Part model, mm, in its own coordinate system. Face numbers are marked on the shaded views. A direction names the side the tool comes from. Coordinates: 2 decimals unless noted, no trailing zeros. Loops run counter-clockwise (first coordinate to the right, second up) from the corner with the lowest first, then second, coordinate; pieces in that order, holes last. Notation, with made-up numbers: M 30,19.25 L 61,19.25 A25 ccw 61,42.25 Z; hole C -12,31.5 d5. An arc over 180 degrees is marked long. Answer as CSV lines item,"result". Start each with the question number.
Autodesk Inventor part; units mm, degrees
ref_plane "YZ Plane" through (0, 0, 0) normal (1, 0, 0) x (0, 1, 0)
ref_plane "XZ Plane" through (0, 0, 0) normal (0, 1, 0) x (-1, 0, 0)
ref_plane "XY Plane" through (0, 0, 0) normal (0, 0, 1) x (1, 0, 0)
sketch "Sketch1" plane through (0, 0, 0) normal (0, 0, 1) x (1, 0, 0)
  line L0 (-107.95, 107.95) -> (107.95, 107.95)
  line L1 (107.95, 107.95) -> (107.95, -107.95)
  line L2 (107.95, -107.95) -> (-107.95, -107.95)
  line L3 (-107.95, -107.95) -> (-107.95, 107.95)
  line L4 (-107.95, -107.95) -> (107.95, 107.95) construction
  point P0 (0, 0)
  point P1 (0, 0)
  dimension "d0" = 215.9
  dimension "d1" = 215.9
extrude "Extrusion1" add sketch "Sketch1" along normal blind 3
sketch "Sketch3" plane through (0, 0, 0) normal (0, 0, -1) x (-1, 0, 0)
  line L0 (256.032, 0) -> (-256.032, 0) construction
  line L1 (0, -256.032) -> (0, 256.032) construction
  line L2 (-101.6, 101.6) -> (101.6, 101.6) construction
  line L3 (-101.6, -101.6) -> (101.6, -101.6) construction
  line L4 (101.6, 101.6) -> (-101.6, -101.6) construction
  line L5 (101.6, -101.6) -> (-101.6, 101.6) construction
  arc A0 (-90.3175, 92.5625) -> (-92.5625, 92.5625) centre (-91.44, 91.44) ccw
  arc A1 (-90.3175, 92.5625) -> (0, 55.1518) centre (0, 182.88) ccw
  line L6 (-91.44, 91.44) -> (0, 182.88) construction
  arc A2 (-92.5625, 92.5625) -> (-92.5625, 90.3175) centre (-91.44, 91.44) ccw
  arc A3 (-55.1518, 0) -> (-92.5625, 90.3175) centre (-182.88, 0) ccw
  arc A4 (92.5625, 92.5625) -> (90.3175, 92.5625) centre (91.44, 91.44) ccw
  arc A5 (0, 55.1518) -> (90.3175, 92.5625) centre (0, 182.88) ccw
  arc A6 (92.5625, 90.3175) -> (55.1518, 0) centre (182.88, 0) ccw
  arc A7 (92.5625, 90.3175) -> (92.5625, 92.5625) centre (91.44, 91.44) ccw
  arc A8 (-92.5625, -92.5625) -> (-90.3175, -92.5625) centre (-91.44, -91.44) ccw
  arc A9 (0, -55.1518) -> (-90.3175, -92.5625) centre (0, -182.88) ccw
  arc A10 (-92.5625, -90.3175) -> (-55.1518, 0) centre (-182.88, 0) ccw
  arc A11 (-92.5625, -90.3175) -> (-92.5625, -92.5625) centre (-91.44, -91.44) ccw
  arc A12 (55.1518, 0) -> (92.5625, -90.3175) centre (182.88, 0) ccw
  arc A13 (90.3175, -92.5625) -> (0, -55.1518) centre (0, -182.88) ccw
  arc A14 (90.3175, -92.5625) -> (92.5625, -92.5625) centre (91.44, -91.44) ccw
  arc A15 (92.5625, -92.5625) -> (92.5625, -90.3175) centre (91.44, -91.44) ccw
  point P0 (0, 0)
  dimension "d168" = 3.175
  dimension "d169" = 91.44
extrude "Extrusion5" cut sketch "Sketch3" against normal blind 0.7
sketch "Sketch6" plane through (0, 0, 0.7) normal (0, 0, -1) x (-1, 0, 0)
  circle A0 centre (0, 0) radius 55.1518
  arc A1 (-90.3175, 92.5625) -> (-92.5625, 90.3175) centre (-91.44, 91.44) ccw
  arc A2 (-92.5625, -90.3175) -> (-92.5625, 90.3175) centre (-182.88, 0) ccw
  arc A3 (-92.5625, -90.3175) -> (-90.3175, -92.5625) centre (-91.44, -91.44) ccw
  arc A4 (90.3175, -92.5625) -> (-90.3175, -92.5625) centre (0, -182.88) ccw
  arc A5 (90.3175, -92.5625) -> (92.5625, -90.3175) centre (91.44, -91.44) ccw
  arc A6 (92.5625, 90.3175) -> (92.5625, -90.3175) centre (182.88, 0) ccw
  arc A7 (92.5625, 90.3175) -> (90.3175, 92.5625) centre (91.44, 91.44) ccw
  arc A8 (-90.3175, 92.5625) -> (90.3175, 92.5625) centre (0, 182.88) ccw
  arc A9 (-90.3175, 92.5625) -> (90.3175, 92.5625) centre (0, 182.88) ccw
  point P0 (0, 0)
extrude "Extrusion6" cut sketch "Sketch6" against normal up to next contours A0
sketch "Sketch11" plane through (0, 0, 3) normal (0, 0, 1) x (1, 0, 0)
  line L0 (-91.44, 91.44) -> (91.44, 91.44) construction
  line L1 (91.44, 91.44) -> (91.44, -91.44) construction
  line L2 (91.44, -91.44) -> (-91.44, -91.44) construction
  line L3 (-91.44, -91.44) -> (-91.44, 91.44) construction
  line L4 (-151.13, 0) -> (151.13, 0) construction
  line L5 (0, -151.13) -> (0, 151.13) construction
  point P0 (0, 0)
  dimension "d170" = 182.88
  dimension "d171" = 182.88
hole "Hole15" at (-91.44, 91.44, 3) at (91.44, 91.44, 3) at (91.44, -91.44, 3) at (-91.44, -91.44, 3) direction (0, 0, -1) diameter 3.175 end through all
sketch "Sketch13" plane through (0, 0, 3) normal (0, 0, 1) x (1, 0, 0)
  line L0 (-91.44, -91.44) -> (91.44, -91.44) construction
  line L1 (91.44, -91.44) -> (91.44, 91.44) construction
  line L2 (91.44, 91.44) -> (-91.44, 91.44) construction
  line L3 (-91.44, 91.44) -> (-91.44, -91.44) construction
  line L4 (-91.44, -91.44) -> (91.44, 91.44) construction
  line L5 (-151.13, 0) -> (151.13, 0) construction
  line L6 (0, -151.13) -> (0, 151.13) construction
  point P0 (0, 0)
  point P1 (0, 0)
  point P2 (-68.58, 91.44)
  point P3 (0, 91.44)
  point P4 (68.58, 91.44)
  point P5 (91.44, 68.58)
  point P6 (91.44, 0)
  point P7 (91.44, -68.58)
  point P8 (68.58, -91.44)
  point P9 (0, -91.44)
  point P10 (-68.58, -91.44)
  point P11 (-91.44, -68.58)
  point P12 (-91.44, 0)
  point P13 (-91.44, 68.58)
  dimension "d302" = 182.88
  dimension "d303" = 182.88
  dimension "d304" = 22.86
  dimension "d305" = 22.86
hole "Hole29" at (-68.58, 91.44, 3) at (0, 91.44, 3) at (68.58, 91.44, 3) at (91.44, 68.58, 3) at (91.44, 0, 3) at (91.44, -68.58, 3) at (68.58, -91.44, 3) at (0, -91.44, 3) at (-68.58, -91.44, 3) at (-91.44, -68.58, 3) at (-91.44, 0, 3) at (-91.44, 68.58, 3) direction (0, 0, -1) diameter 4.4958 end through all
sketch "Sketch14" plane through (0, 0, 3) normal (0, 0, 1) x (1, 0, 0)
  circle A0 centre (0, 0) radius 55.1518
  line L0 (0, -151.13) -> (0, 151.13) construction
  circle A1 centre (0, 55.1518) radius 1.5875
  point P0 (0, 0)
  dimension "d313" = 3.175
extrude "Extrusion9" cut sketch "Sketch14" against normal through all contours A1 A0 | A0 A1 picked at (0.0632, 54.6247) picked at (0.0603, 55.6758)
equation "\"d1\" = d0"
properties part number "J002446_1" material "UHMW, WHITE"
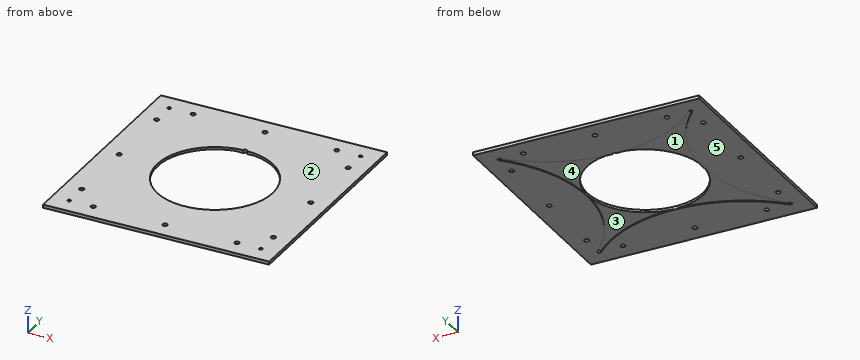
Q1. Slice it at B-B, the plane x = -10. Write the cut outline in (y, z).
Q2. Slice it at C-C, the plane x = 21. Write the cut outline in (y, z), and give its area (3 significant figures).
Q3. Two-plate mould, pull along X, no slides. Class the marked faces 3, 4 and 5: +X half, -X half, draft (parallel to the pull), parting line (faces both ways), or undercut.
Q4. Slice it at A-A, the plane z = 2.1. State how many separate pieces and enclosed holes the cut face has, and give its area (3 significant figures).
Q5. Tool access for the marked faces 1 and 2: list every direction of +Z, -Z, +X, -X, +Y, -Y with a clear straight run to the whole face (end or side of a thin tool).
Q6. Wall check: L1, parallel to X at y = 0, z = 1.1; L2, parallel to X at y = 91.44, z = 2.15. Give the ranges that are in metal, low to high.
Solved:
1,outline,"M -107.95,0 L -55.54,0 L -55.54,0.7 L -54.24,0.7 L -54.24,3 L -107.95,3 Z; M 54.24,0.7 L 55.54,0.7 L 55.54,0 L 107.95,0 L 107.95,3 L 54.24,3 Z"
2,outline,"M -107.95,0 L -56.89,0 L -56.89,0.7 L -51,0.7 L -51,3 L -107.95,3 Z; M 51,0.7 L 56.89,0.7 L 56.89,0 L 107.95,0 L 107.95,3 L 51,3 Z"
2,area,"333 mm2"
3,face 3,"undercut"
3,face 4,"undercut"
3,face 5,"draft"
4,separate pieces,"1"
4,enclosed holes,"17"
4,area,"36,800 mm2"
5,face 1,"-Z"
5,face 2,"+Z, +X, -X, +Y, -Y"
6,L1,"x = -107.95 to -93.69, -89.19 to -55.15, 55.15 to 89.19, 93.69 to 107.95"
6,L2,"x = -107.95 to -93.03, -89.85 to -70.83, -66.33 to -2.25, 2.25 to 66.33, 70.83 to 89.85, 93.03 to 107.95"
